```python
from build123d import *

# Parameters (mm, degrees)
PAD_DEPTH       = 40
POCKET_DEPTH    = 35
SKETCH002_R     = 1.25
SKETCH002_W     = 27
SKETCH002_H     = 4
POCKET001_DEPTH = 10
SKETCH003_R     = 2
HOLE_DEPTH      = 5
HOLE_TIPS_R     = 2
SKETCH004_R     = 5
POCKET002_DEPTH = 1
SKETCH009_R     = 1.9
POCKET005_DEPTH = 100


with BuildPart() as part:
    # Sketch → Pad (new body)
    with BuildSketch(Plane.XY):
        with BuildLine():
            ThreePointArc((-35, 25), (-38.535534, 23.535534), (-40, 20))
            Line((-40, -20), (-40, 20))
            ThreePointArc((-40, -20), (-38.535534, -23.535534), (-35, -25))
            Line((35, -25), (-35, -25))
            ThreePointArc((35, -25), (38.535534, -23.535534), (40, -20))
            Line((40, 20), (40, -20))
            ThreePointArc((40, 20), (38.535534, 23.535534), (35, 25))
            Line((-35, 25), (35, 25))
        make_face()
    extrude(amount=PAD_DEPTH)

    # Sketch001 (on Face10 of Pad) → Pocket (cut)
    with BuildSketch(Plane.XY.offset(40)):
        Polygon((-32.5, 14.82538), (-29.82538, 17.5), (29.82538, 17.5), (32.5, 14.82538), (32.5, -14.82538), (29.82538, -17.5), (-29.82538, -17.5), (-32.5, -14.82538), align=None)
    extrude(amount=-POCKET_DEPTH, mode=Mode.SUBTRACT)

    # Sketch002 (on Face4 of Pocket) → Pocket001 (cut)
    with BuildSketch(Plane(origin=(0, 0, 0), x_dir=(1, 0, 0), z_dir=(0, 0, -1))):
        with Locations((-12, 12)):
            Circle(SKETCH002_R)
        with Locations((12, 12)):
            Circle(SKETCH002_R)
        with Locations((-12, -12)):
            Circle(SKETCH002_R)
        with Locations((12, -12)):
            Circle(SKETCH002_R)
        Rectangle(SKETCH002_W, SKETCH002_H)
        with Locations((0, 5)):
            Rectangle(SKETCH002_W, SKETCH002_H)
        with Locations((0, -5)):
            Rectangle(SKETCH002_W, SKETCH002_H)
        Polygon((-13.5, 8), (-6.180741, 13.125), (6.180741, 13.125), (13.5, 8), align=None)
        Polygon((-13.5, -8), (13.5, -8), (6.180741, -13.125), (-6.180741, -13.125), align=None)
    extrude(amount=-POCKET001_DEPTH, mode=Mode.SUBTRACT)

    # Sketch003 (on Face5 of Pocket001) → Hole (cut)
    with BuildSketch(Plane.XY.offset(40)):
        with Locations((-35, 20)):
            Circle(SKETCH003_R)
        with Locations((35, 20)):
            Circle(SKETCH003_R)
        with Locations((35, -20)):
            Circle(SKETCH003_R)
        with Locations((-35, -20)):
            Circle(SKETCH003_R)
    extrude(amount=-HOLE_DEPTH, mode=Mode.SUBTRACT)

    # Hole tips → Hole tip 1 section 0
    with BuildSketch(Plane.XY.offset(35), mode=Mode.PRIVATE) as hole_tip_1_s0:
        with Locations((-35, 20)):
            Circle(HOLE_TIPS_R)
    loft([hole_tip_1_s0.sketch, Vertex(-35, 20, 33.798279)], mode=Mode.SUBTRACT)

    # Hole tips → Hole tip 2 section 0
    with BuildSketch(Plane.XY.offset(35), mode=Mode.PRIVATE) as hole_tip_2_s0:
        with Locations((35, 20)):
            Circle(HOLE_TIPS_R)
    loft([hole_tip_2_s0.sketch, Vertex(35, 20, 33.798279)], mode=Mode.SUBTRACT)

    # Hole tips → Hole tip 3 section 0
    with BuildSketch(Plane.XY.offset(35), mode=Mode.PRIVATE) as hole_tip_3_s0:
        with Locations((35, -20)):
            Circle(HOLE_TIPS_R)
    loft([hole_tip_3_s0.sketch, Vertex(35, -20, 33.798279)], mode=Mode.SUBTRACT)

    # Hole tips → Hole tip 4 section 0
    with BuildSketch(Plane.XY.offset(35), mode=Mode.PRIVATE) as hole_tip_4_s0:
        with Locations((-35, -20)):
            Circle(HOLE_TIPS_R)
    loft([hole_tip_4_s0.sketch, Vertex(-35, -20, 33.798279)], mode=Mode.SUBTRACT)

    # Sketch004 (on Face4 of Hole) → Pocket002 (cut)
    with BuildSketch(Plane(origin=(0, 0, 0), x_dir=(1, 0, 0), z_dir=(0, 0, -1))):
        with Locations((-30, 15)):
            Circle(SKETCH004_R)
        with Locations((-30, -15)):
            Circle(SKETCH004_R)
        with Locations((30, 15)):
            Circle(SKETCH004_R)
        with Locations((30, -15)):
            Circle(SKETCH004_R)
    extrude(amount=-POCKET002_DEPTH, mode=Mode.SUBTRACT)

    # Sketch009 (on Face9 of Hole) → Pocket005 (cut)
    with BuildSketch(Plane(origin=(-40, 0, 0), x_dir=(0, -1, 0), z_dir=(-1, 0, 0))):
        with Locations((0, 30)):
            Circle(SKETCH009_R)
    extrude(amount=-POCKET005_DEPTH, mode=Mode.SUBTRACT)


solid = part.part
```
Geometry: final body of the model. Coordinates: model frame, mm. A direction names the side the tool comes from. Coordinates: 2 decimals unless noted, no trailing zeros. Order: outer loops, then holes, each group sorted by start corner. A loop starts at its lowest first (then second) coordinate and runs counter-clockwise, first axis right, second up.
Item 1: Access query for faces 4 (the face through (36.908, 20.601, 37.535)), 5 (the face through (-34, -12, 0.5)), 6 (the face through (13.5, -5, 2)). Directions: +Z, -Z, +X, -X, +Y, -Y. A direction counts if a zero-diameter tool reaches every point of the face in a straight line with its end or side. Return the directions, or none.
Answer:
face 4: +Z
face 5: -Z
face 6: +Z, -Z
Item 2: Material intervals for line 1 along X through (y, z) = (-1.5, 13); line 2 along Y through (x, z) = (-20.5, 7); line 3 along Z through (x, y) = (-37, 0), sorted ascending.
Answer:
line 1: x = -40 to -32.5, 32.5 to 40
line 2: y = -25 to -17.5, 17.5 to 25
line 3: z = 0 to 28.1, 31.9 to 40
Item 3: Section query A-A (z = 37). Output: boundary loops of the cut face in (x, y).
Answer:
outline: (-40, -20) arc R5 ccw to (-35, -25) - (35, -25) arc R5 ccw to (40, -20) - (40, 20) arc R5 ccw to (35, 25) - (-35, 25) arc R5 ccw to (-40, 20) - close; hole circle Ø4 at (-35, -20); hole circle Ø4 at (-35, 20); hole (-32.5, -14.83) - (-29.83, -17.5) - (29.83, -17.5) - (32.5, -14.83) - (32.5, 14.83) - (29.83, 17.5) - (-29.83, 17.5) - (-32.5, 14.83) - close; hole circle Ø4 at (35, -20); hole circle Ø4 at (35, 20)
Item 4: Section query B-B (y = 0). Output: boundary loops of the cut face in (x, z), then the cut area to 3 significant figures.
Answer:
outline: (-40, 0) - (-13.5, 0) - (-13.5, 5) - (-32.5, 5) - (-32.5, 28.1) - (-40, 28.1) - close; (-40, 31.9) - (-32.5, 31.9) - (-32.5, 40) - (-40, 40) - close; (13.5, 0) - (40, 0) - (40, 28.1) - (32.5, 28.1) - (32.5, 5) - (13.5, 5) - close; (32.5, 31.9) - (40, 31.9) - (40, 40) - (32.5, 40) - close
area: 733 mm2
Item 5: Section query C-C (z = 23.5). Output: boundary loops of the cut face in (x, y).
Answer:
outline: (-40, -20) arc R5 ccw to (-35, -25) - (35, -25) arc R5 ccw to (40, -20) - (40, 20) arc R5 ccw to (35, 25) - (-35, 25) arc R5 ccw to (-40, 20) - close; hole (-32.5, -14.83) - (-29.83, -17.5) - (29.83, -17.5) - (32.5, -14.83) - (32.5, 14.83) - (29.83, 17.5) - (-29.83, 17.5) - (-32.5, 14.83) - close
Item 6: Draft query along X for faces 1 (the face through (-38, 24, 20)), 2 (the face through (31.144, 16.181, 22.745)), 3 (the face through (0, -25, 20)). Return one class per face: released by +X, released by -X, zero draft, split by the parting line, or undercut.
Answer:
face 1: released by -X
face 2: undercut
face 3: zero draft
Item 7: Section query D-D (x = -9.5). Output: boundary loops of the cut face in (y, z).
Answer:
outline: (-25, 0) - (-10.8, 0) - (-10.8, 5) - (-17.5, 5) - (-17.5, 40) - (-25, 40) - close; (-8, 0) - (-7, 0) - (-7, 5) - (-8, 5) - close; (-3, 0) - (-2, 0) - (-2, 5) - (-3, 5) - close; (2, 0) - (3, 0) - (3, 5) - (2, 5) - close; (7, 0) - (8, 0) - (8, 5) - (7, 5) - close; (10.8, 0) - (25, 0) - (25, 40) - (17.5, 40) - (17.5, 5) - (10.8, 5) - close
Item 8: Contact query for flat-ended pins moving along their axis: P1, Ø10.5, axis at x = -10.5, y = 2.5, coming from the +Z side; P2, Ø3.5, axis at x = 35, y = -20, coming from the +Z side; P3, Ø9, axis at x = 30, y = -15, coming from the -Z side. Output: stop coordinate, or through.
Answer:
P1: stops at z = 5
P2: stops at z = 34.85
P3: stops at z = 1
